from build123d import *

# Parameters (mm, degrees)
F0_R        = 2.5
F0_R_2      = 23.5
F0_R_3      = 19.5
F1_DEPTH    = 3
F2_DEPTH    = 2.5
F3_T1_DEPTH = 32.6645215065


# Not quite as in the source:
# - a fillet or chamfer that OpenCascade refuses, or shapes differently, is made with other operations: its cross-section is extruded or revolved along the edge and cut away or added


with BuildPart() as f1:
    # F0 (on Top) → F1 (new body)
    with BuildSketch(Plane.XY):
        with BuildLine():
            Line((-20.3162496539, -28.5), (20.3162496539, -28.5))
            ThreePointArc((20.3162496539, -28.5), (24.7487373415, -24.7487373415), (28.5, -20.3162496539))
            Line((28.5, -20.3162496539), (28.5, 20.3162496539))
            ThreePointArc((28.5, 20.3162496539), (24.7487373415, 24.7487373415), (20.3162496539, 28.5))
            Line((20.3162496539, 28.5), (-20.3162496539, 28.5))
            ThreePointArc((-20.3162496539, 28.5), (-24.7487373415, 24.7487373415), (-28.5, 20.3162496539))
            Line((-28.5, 20.3162496539), (-28.5, -20.3162496539))
            ThreePointArc((-28.5, -20.3162496539), (-24.7487373415, -24.7487373415), (-20.3162496539, -28.5))
        make_face()
        with Locations((-21.5, -21.5)):
            Circle(F0_R, mode=Mode.SUBTRACT)
        with Locations((21.5, -21.5)):
            Circle(F0_R, mode=Mode.SUBTRACT)
        with Locations((-21.5, 21.5)):
            Circle(F0_R, mode=Mode.SUBTRACT)
        Circle(F0_R_2, mode=Mode.SUBTRACT)
        with Locations((21.5, 21.5)):
            Circle(F0_R, mode=Mode.SUBTRACT)
        Circle(F0_R_2)
        Circle(F0_R_3, mode=Mode.SUBTRACT)
    extrude(amount=F1_DEPTH)

    # F0 (on Top) → F2 (join)
    with BuildSketch(Plane.XY):
        Circle(F0_R_2)
        Circle(F0_R_3, mode=Mode.SUBTRACT)
    extrude(amount=F2_DEPTH)

    # F3: fillet of radius 13 on 8 edges, made by hand

    # F3_s2 → F3_t1 (cut)
    with BuildSketch(Plane.XY.offset(-14.8322607533)):
        with BuildLine():
            ThreePointArc((-28.5, 15.612494996), (-27.5014203705, 20.6090847421), (-24.6590909091, 24.8380602209))
            ThreePointArc((-24.6590909091, 24.8380602209), (-26.675530534, 22.6586864299), (-28.5, 20.3162496539))
            Line((-28.5, 20.3162496539), (-28.5, 15.612494996))
        make_face()
        with BuildLine():
            ThreePointArc((-24.8380602209, 24.6590909091), (-20.6090847421, 27.5014203705), (-15.612494996, 28.5))
            Line((-15.612494996, 28.5), (-20.3162496539, 28.5))
            ThreePointArc((-20.3162496539, 28.5), (-22.6586864299, 26.675530534), (-24.8380602209, 24.6590909091))
        make_face()
        with BuildLine():
            ThreePointArc((15.612494996, 28.5), (20.6090847421, 27.5014203705), (24.8380602209, 24.6590909091))
            ThreePointArc((24.8380602209, 24.6590909091), (22.6586864299, 26.675530534), (20.3162496539, 28.5))
            Line((20.3162496539, 28.5), (15.612494996, 28.5))
        make_face()
        with BuildLine():
            ThreePointArc((24.6590909091, 24.8380602209), (27.5014203705, 20.6090847421), (28.5, 15.612494996))
            Line((28.5, 15.612494996), (28.5, 20.3162496539))
            ThreePointArc((28.5, 20.3162496539), (26.675530534, 22.6586864299), (24.6590909091, 24.8380602209))
        make_face()
        with BuildLine():
            ThreePointArc((28.5, -15.612494996), (27.5014203705, -20.6090847421), (24.6590909091, -24.8380602209))
            ThreePointArc((24.6590909091, -24.8380602209), (26.675530534, -22.6586864299), (28.5, -20.3162496539))
            Line((28.5, -20.3162496539), (28.5, -15.612494996))
        make_face()
        with BuildLine():
            ThreePointArc((24.8380602209, -24.6590909091), (20.6090847421, -27.5014203705), (15.612494996, -28.5))
            Line((15.612494996, -28.5), (20.3162496539, -28.5))
            ThreePointArc((20.3162496539, -28.5), (22.6586864299, -26.675530534), (24.8380602209, -24.6590909091))
        make_face()
        with BuildLine():
            ThreePointArc((-24.8380602209, -24.6590909091), (-20.6090847421, -27.5014203705), (-15.612494996, -28.5))
            Line((-15.612494996, -28.5), (-20.3162496539, -28.5))
            ThreePointArc((-20.3162496539, -28.5), (-22.6586864299, -26.675530534), (-24.8380602209, -24.6590909091))
        make_face()
        with BuildLine():
            ThreePointArc((-24.6590909091, -24.8380602209), (-27.5014203705, -20.6090847421), (-28.5, -15.612494996))
            Line((-28.5, -15.612494996), (-28.5, -20.3162496539))
            ThreePointArc((-28.5, -20.3162496539), (-26.675530534, -22.6586864299), (-24.6590909091, -24.8380602209))
        make_face()
    extrude(amount=F3_T1_DEPTH, mode=Mode.SUBTRACT)

    # F4: chamfer of 2.5 on 4 edges, made by hand

    # F4_s1 → F4_t2 (revolve, cut)
    with BuildSketch(Plane.XZ.offset(-21.5)):
        Polygon((-16.5, 3), (-19, 0.5), (-19, 3), align=None)
    revolve(axis=Axis((-21.5, 21.5, 3), (0, 0, 1)), mode=Mode.SUBTRACT)

    # F4_s3 → F4_t4 (revolve, cut)
    with BuildSketch(Plane.XZ.offset(-21.5)):
        Polygon((26.5, 3), (24, 0.5), (24, 3), align=None)
    revolve(axis=Axis((21.5, 21.5, 3), (0, 0, 1)), mode=Mode.SUBTRACT)

    # F4_s5 → F4_t6 (revolve, cut)
    with BuildSketch(Plane.XZ.offset(21.5)):
        Polygon((26.5, 3), (24, 0.5), (24, 3), align=None)
    revolve(axis=Axis((21.5, -21.5, 3), (0, 0, 1)), mode=Mode.SUBTRACT)

    # F4_s7 → F4_t8 (revolve, cut)
    with BuildSketch(Plane.XZ.offset(21.5)):
        Polygon((-16.5, 3), (-19, 0.5), (-19, 3), align=None)
    revolve(axis=Axis((-21.5, -21.5, 3), (0, 0, 1)), mode=Mode.SUBTRACT)


solid = f1.part
The model under review builds one solid part; all positions refer to its coordinate system, in mm. Give positions to 0.01 mm unless a question says otherwise; leave off trailing zeros. Write each loop counter-clockwise with the first axis right and the second up, starting at its lowest first coordinate (ties: lowest second). Pieces come first, ordered by that corner, then holes.
1. Add section D-D, the plane x = -21.5. Write out the cut boundary in (y, z).
2. Add section B-B, the plane x = 0. Write out the cut boundary in (y, z).
3. Wall thickness on L1, parallel to Y at x = 21.5, z = 0.35; L2, parallel to Y at x = 20, z = 0.6; L3, parallel to X at y = 0.5, z = 2.85: over which ranges is each line inside the solid? List them lowest first.
4. Draft analysis for pull direction X (two halves, no side actions). For faces 1 (the flat face through (-7, 19, 3)), 2 (the conical face through (-20.09, -19.29, 0.62)), 3 (the flat face through (28.5, 0, 1)), state which applies: +X half, -X half, draft (parallel to the pull), parting line (faces both ways), or undercut.
5. Add section A-A, the plane z = 1.5. Write out the cut boundary in (x, y), plus the area to 3 significant figures.
6. For P1, Ø8, axis at x = -21.5, y = -21.5, coming from the +Z side; P2, Ø6, axis at x = -21.5, y = 21.5, coming from the +Z side; P3, Ø6.5, axis at x = 21.5, y = 21.5, coming from the +Z side; P4, Ø6.5, axis at x = 21.5, y = -21.5, coming from the -Z side, all flat-tipped, find the tip position at first contact; note any pin that passes through.
Worked answers:
1. outline: (-27.09, 0) - (-24, 0) - (-24, 0.5) - (-26.5, 3) - (-27.09, 3) - close; (-19, 0) - (19, 0) - (19, 0.5) - (16.5, 3) - (-16.5, 3) - (-19, 0.5) - close; (24, 0) - (27.09, 0) - (27.09, 3) - (26.5, 3) - (24, 0.5) - close
2. outline: (-28.5, 0) - (-19.5, 0) - (-19.5, 3) - (-28.5, 3) - close; (19.5, 0) - (28.5, 0) - (28.5, 3) - (19.5, 3) - close
3. L1: y = -27.09 to -24, -19 to 19, 24 to 27.09
3. L2: y = -27.74 to -23.62, -19.38 to 19.38, 23.62 to 27.74
3. L3: x = -28.5 to -19.49, 19.49 to 28.5
4. face 1: draft
4. face 2: undercut
4. face 3: +X half
5. outline: (-28.5, -15.61) arc R13 ccw to (-24.75, -24.75) arc R13 ccw to (-15.61, -28.5) - (15.61, -28.5) arc R13 ccw to (24.75, -24.75) arc R13 ccw to (28.5, -15.61) - (28.5, 15.61) arc R13 ccw to (24.75, 24.75) arc R13 ccw to (15.61, 28.5) - (-15.61, 28.5) arc R13 ccw to (-24.75, 24.75) arc R13 ccw to (-28.5, 15.61) - close; hole circle Ø7 at (-21.5, -21.5); hole circle Ø7 at (-21.5, 21.5); hole circle Ø39 at (0, 0); hole circle Ø7 at (21.5, -21.5); hole circle Ø7 at (21.5, 21.5)
5. area: 1,760 mm2
6. P1: stops at z = 2
6. P2: stops at z = 1
6. P3: stops at z = 1.25
6. P4: stops at z = 0
